Can you work these out from the model? Positions are in its coordinate system, mm. A direction names the side the tool comes from. Give positions to 0.01 mm unless a question says otherwise; leave off trailing zeros. Order: outer loops, then holes, each group sorted by start corner. A loop starts at its lowest first (then second) coordinate and runs counter-clockwise, first axis right, second up. Notation, with made-up numbers: (9.25, 59) - (20.25, 59) arc R33 cw to (20.25, 89) - close; hole circle Ø2 at (56, 6). An arc over 180 degrees is marked (long way). Answer as a JSON object with one key per item and string values.
Autodesk Inventor part; units mm, degrees
ref_plane "YZ Plane" through (0, 0, 0) normal (1, 0, 0) x (0, 1, 0)
ref_plane "XZ Plane" through (0, 0, 0) normal (0, 1, 0) x (-1, 0, 0)
ref_plane "XY Plane" through (0, 0, 0) normal (0, 0, 1) x (1, 0, 0)
sketch "Sketch1" plane through (0, 0, 0) normal (0, 1, 0) x (-1, 0, 0)
  circle A0 centre (0, 0) radius 4.8
  dimension "d0" = 9.6
extrude "Extrusion1" add sketch "Sketch1" along normal blind 162
sketch "Sketch2" plane through (0, 162, 0) normal (0, 1, 0) x (1, 0, 0)
  line L0 (-3.8312, -2.1) -> (3.8312, -2.1)
  line L1 (3.8312, -2.1) -> (3.8312, 2.1)
  line L2 (3.8312, 2.1) -> (-3.8312, 2.1)
  line L3 (-3.8312, 2.1) -> (-3.8312, -2.1)
  line L4 (-3.8312, -2.1) -> (3.8312, 2.1) construction
  line L5 (3.8312, -2.1) -> (-3.8312, 2.1) construction
  arc A0 (-3.8312, 2.1) -> (-3.8312, -2.1) centre (-0.4025, 0) ccw
  line L6 (-4.4232, 0) -> (-3.8312, 0)
  line L7 (3.8312, 0) -> (4.4232, 0)
  arc A1 (3.8312, -2.1) -> (3.8312, 2.1) centre (0.4025, 0) ccw
  circle A2 centre (0, 0) radius 4.8
  line L8 (-4.8, 0) -> (-4.4232, 0)
  line L9 (4.4232, 0) -> (4.8, 0)
  dimension "d3" = 0.592
  dimension "d6" = 4.2
extrude "Extrusion2" cut sketch "Sketch2" against normal blind 7 contours L3 L2 L1 L0 | A0 L6 L3 | L1 L7 A1 | L6 A0 L3 | L1 A1 L7
properties part number "Lifting Shaft"
Q1. If we section it at A-A, the plane z = 0: Please give me the cut outline in (x, y).
Recorded:
{"outline": "(-4.8, 0) - (4.8, 0) - (4.8, 162) - (4.42, 162) - (4.42, 155) - (-4.42, 155) - (-4.42, 162) - (-4.8, 162) - close"}
Q2. If we section it at B-B, the plane x = 0: Please give me the cut outline in (y, z).
Recorded:
{"outline": "(0, -4.8) - (162, -4.8) - (162, -2.1) - (155, -2.1) - (155, 2.1) - (162, 2.1) - (162, 4.8) - (0, 4.8) - close"}
Q3. I need wall thicknesses on L1, parallel to X at y = 153, z = -0.25; L2, parallel to Y at x = -2, z = 0.25; L3, parallel to Z at x = 2, y = 93. Which ranges of each line are inside material? Lowest first, please.
Recorded:
{"L1": "x = -4.79 to 4.79", "L2": "y = 0 to 155", "L3": "z = -4.36 to 4.36"}
Q4. If we section it at C-C, the plane y = 141: Please give me the cut outline in (x, z), then the cut area to 3 significant figures.
Recorded:
{"outline": "circle Ø9.6 at (0, 0)", "area": "72.4 mm^2"}
Q5. Which directions (+Z, -Z, +X, -X, +Y, -Y) give clear straight access to the entire face, cutting with the end or side of a thin tool? Please do faces 4 (the face through (0, 159, 2.1)), 5 (the face through (0, 162, 3)).
Recorded:
{"face 4": "+Y", "face 5": "+Z, -Z, +X, -X, +Y"}
Q6. We'd pull the mould along Z, two halves only. Please class faces 1 (the face through (-2.58, 79.87, -4.05)), 2 (the face through (0, 159, -2.1)), 3 (the face through (0, 0, 0)): released by +Z, released by -Z, zero draft, split by the parting line, or undercut.
Recorded:
{"face 1": "split by the parting line", "face 2": "undercut", "face 3": "zero draft"}
Q7. I'm going to push flat-ended pins straight in: pin 1 Ø1 at (x, y) = (1, 118.5) entering from +Z; pin 2 Ø1 at (x, y) = (1, 56.5) entering from -Z. Where does each tip first touch, or does it pass through?
Recorded:
{"pin 1": "stops at z = 4.77", "pin 2": "stops at z = -4.77"}
